CAD build for the part. Positions are in the model's coordinates, mm. Face numbers are marked on the shaded views. A direction names the side the tool comes from. Round coordinates to 2 decimals unless told otherwise and drop trailing zeros. Loops run counter-clockwise (first coordinate to the right, second up) from the corner with the lowest first, then second, coordinate; pieces in that order, holes last.
Autodesk Inventor part; units mm, degrees
ref_plane "Work Plane1" through (17.4207, 0, 0) normal (0, 0, -1) x (-1, 0, 0)
ref_plane "YZ Plane" through (0, 0, 0) normal (1, 0, 0) x (0, 1, 0)
ref_plane "XZ Plane" through (0, 0, 0) normal (0, 1, 0) x (-1, 0, 0)
sketch "Эскиз1" plane through (0, 0, 0) normal (0, 0, 1) x (1, 0, 0)
  line L0 (-1.2035, 0) -> (6.0339, 0)
  line L1 (2.5231, 4) -> (1.9063, 5.3226)
  line L2 (2.5231, 4) -> (5, 4) construction
  line L3 (5, 4) -> (5, 0) construction
  arc A0 (1.9063, 5.3226) -> (0, 4.9) centre (1, 4.9) ccw
  line L4 (2.5231, 4) -> (2.5231, 0)
  line L5 (0, -1.2175) -> (0, 7.3051)
  point P0 (0, 0)
  dimension "d2" = 8
  dimension "d4" = 11.8
  dimension "d5" = 1
  dimension "d15" = 5
  dimension "d16" = 25
revolve "Кольцо" add sketch "Эскиз1" angle 360 about axis through (-10, 0, 0) along (1, 0, 0)
sketch "Эскиз2" plane through (0, 0, 0) normal (-1, 0, 0) x (0, 0, 1)
  circle A0 centre (0, 0) radius 4.9
  line L0 (-4, -2.3094) -> (-4, 2.3094)
  line L1 (-4, 2.3094) -> (0, 4.6188)
  line L2 (0, 4.6188) -> (4, 2.3094)
  line L3 (4, 2.3094) -> (4, -2.3094)
  line L4 (4, -2.3094) -> (0, -4.6188)
  line L5 (0, -4.6188) -> (-4, -2.3094)
  circle A1 centre (0, 0) radius 4.9
  dimension "d6" = 9.2376
extrude "Базовый элемент" add sketch "Эскиз2" against normal blind 5 contours L0 L1 L2 L3 L4 L5
sketch "Эскиз3" plane through (0, 0, 0) normal (0, 0, 1) x (1, 0, 0)
  line L0 (2.2345, 4.6188) -> (5, 4.6188)
  line L1 (5, 2.3094) -> (5, 4.6188)
  line L2 (0, -4.9) -> (0, 4.9)
  line L3 (-1, 0) -> (6, 0)
  line L4 (4.8342, 4.6188) -> (5, 4)
  dimension "d10" = 15
  dimension "d11" = 8
revolve "Фаска1" cut sketch "Эскиз3" angle 360 about axis through (-10, 0, 0) along (1, 0, 0)
sketch "Эскиз4" plane through (0, 0, 0) normal (-1, 0, 0) x (0, 0, 1)
  circle A0 centre (0, 0) radius 4.9
hole "Резьба" at (0, 0, 0) direction (1, 0, 0) diameter 4.134 end through all
chamfer "Фаска2" distance 0.433 angle 30 1 edges at (0, 0, -2.067) measured on face at (0, 3.9032, -0.4739)
ref_plane "Work Plane1" through (17.4207, 0, 0) normal (0, 0, -1) x (-1, 0, 0)
chamfer "Фаска3" distance 0.433 angle 45 1 edges at (5, 0, -2.067)
equation "\"d6\" = 1.1547 * SW"
equation "\"d7\" = KOH"
equation "\"d12\" = -0.5 * GD1 + 0.5 * NND"
equation "\"d46\" = -0.5 * GD1 + 0.5 * NND"
equation "\"d51\" = -0.5 * GD1 + 0.5 * NND"
equation "\"d2\" = SW"
equation "\"d4\" = LADI"
equation "\"d5\" = PHH"
equation "\"d15\" = KOH"
equation "\"d16\" = KEWI"
equation "\"d10\" = ANG1"
equation "\"d11\" = SW0"
equation "\"ANG1\" = 15deg"
equation "\"KEWI\" = 25deg"
equation "\"NND\" = 5"
equation "\"LADI\" = 11.8"
equation "\"SW\" = 8"
equation "\"PHH\" = RR"
equation "\"KOH\" = NND"
equation "\"SW0\" = SW"
equation "\"d1\" = LADI"
equation "\"d3\" = PHH"
equation "\"GUL\" = 0.541266 * PTC"
equation "\"RR\" = 1"
equation "\"THREADDIA\" = 5"
equation "\"TOA\" = 30deg"
equation "\"PTC\" = 0.8"
equation "\"GAL\" = 0.541266 * PTC"
equation "\"E0\" = 1.155 * SW"
properties part number "DIN 6923 - M5" material "Сталь, мягкая"
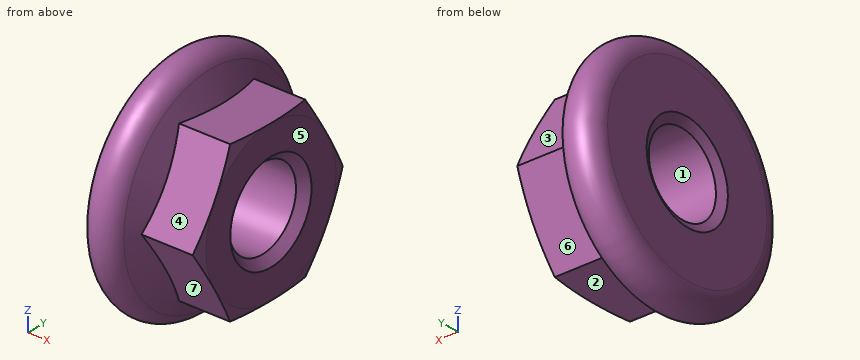
Item 1: Cut at B-B (x = 1.4). List the corners of the cut face in (y, z), plus the area to 3 significant figures.
Verdict:
outline: circle Ø11.63 at (0, 0); hole circle Ø4.13 at (0, 0)
area: 92.9 mm2
Item 2: 3-axis set-ups, long thin cutter, end or side, ignore diameter. For the marked faces 4, 5, 6 and 7: which of +Z, -Z, +X, -X, +Y, -Y reach the whole face in a straight line?
Verdict:
face 4: +Z, +X, -Y
face 5: +Z, -Z, +X, +Y, -Y
face 6: -Z, +X, +Y
face 7: -Z, +X, -Y
Item 3: Wall check: L1, parallel to Y at x = 0.85, z = -0.5; L2, parallel to Z at x = 2.65, y = 0; L3, parallel to Z at x = 1.4, y = -1. Give the ranges that are in metal, low to high.
Verdict:
L1: y = -5.87 to -2.01, 2.01 to 5.87
L2: z = -4 to -2.07, 2.07 to 4
L3: z = -5.73 to -1.81, 1.81 to 5.73
Item 4: Cut at C-C (x = 2.05). List the corners of the cut face in (y, z), plus the area to 3 significant figures.
Verdict:
outline: circle Ø10.03 at (0, 0); hole circle Ø4.13 at (0, 0)
area: 65.6 mm2
Item 5: Mould opens along Y. For the marked faces 1, 2 and 3 say: released by +Y, released by -Y, zero draft, split by the parting line, or undercut.
Verdict:
face 1: undercut
face 2: zero draft
face 3: released by +Y
Item 6: Cut at A-A (x = 3.3). List the corners of the cut face in (y, z), plus the area to 3 significant figures.
Verdict:
outline: (-4.62, 0) - (-2.31, -4) - (2.31, -4) - (4.62, 0) - (2.31, 4) - (-2.31, 4) - close; hole circle Ø4.13 at (0, 0)
area: 42.0 mm2
Item 7: Flat gauge pins, fed straight in: P1, Ø1, axis at x = 1, y = -3, coming from the -Z side; P2, Ø0.8, axis at x = 3, y = 0, coming from the -Z side; P3, Ø0.8, axis at x = 4, y = 0, coming from the +Z side. Where does each tip first touch, or does it go through?
Verdict:
P1: stops at z = -5.34
P2: stops at z = -4
P3: stops at z = 4
